Design review of the part built by this model. Coordinates are the model's own, in mm. Face numbers are marked on the shaded views. A direction names the side the tool comes from. Give positions to 0.01 mm unless a question says otherwise; leave off trailing zeros. Write each loop counter-clockwise with the first axis right and the second up, starting at its lowest first coordinate (ties: lowest second). Pieces come first, ordered by that corner, then holes. Notation, with made-up numbers: (34, 17) -> (81, 17) arc R31 cw to (81, 46) -> close; hole circle Ø9 at (53.5, 12.25). An arc over 180 degrees is marked (long way). Answer as a JSON object with one key per item and string values.
```python
from build123d import *

# Parameters (mm, degrees)
ESQUISSE1_R             = 3.65
BOSS_EXTRU_1_DEPTH      = 7.5
ESQUISSE2_R             = 1.45
ENL_V_MAT_EXTRU_1_DEPTH = 7.2
ENL_V_MAT_EXTRU_1_DRAFT = -0.5
ESQUISSE3_R             = 2.1
BOSS_EXTRU_2_DEPTH      = 5
BOSS_EXTRU_2_DRAFT      = -1
CONG_2_R                = 0.5


with BuildPart() as part:
    # Esquisse1 → Boss.-Extru.1 (new body)
    with BuildSketch(Plane.XY):
        Circle(ESQUISSE1_R)
    extrude(amount=BOSS_EXTRU_1_DEPTH)


with BuildPart() as enl_v_mat_extru_1_tool:
    # Esquisse2 → Enlèv. mat.-Extru.1 (with draft: the straight prism first)
    with BuildSketch(Plane(origin=(4, 0, 0), x_dir=(0, 0, -1), z_dir=(1, 0, 0))):
        with Locations((-3, 0)):
            Circle(ESQUISSE2_R)
    extrude(amount=-ENL_V_MAT_EXTRU_1_DEPTH)
    # Enlèv. mat.-Extru.1: the draft: its side faces are tilted about the plane it starts from
    enl_v_mat_extru_1_sides = [enl_v_mat_extru_1_tool.faces().sort_by_distance(p)[0] for p in [
        (0.4, 0, 4.45),
    ]]
    draft(enl_v_mat_extru_1_sides, Plane(origin=(4, 0, 0), x_dir=(0, 0, -1), z_dir=(1, 0, 0)), ENL_V_MAT_EXTRU_1_DRAFT)


with BuildPart() as part_1:
    add(part.part)

    # Enlèv. mat.-Extru.1: cut by enl_v_mat_extru_1_tool
    add(enl_v_mat_extru_1_tool.part, mode=Mode.SUBTRACT)


with BuildPart() as boss_extru_2_tool:
    # Esquisse3 → Boss.-Extru.2 (with draft: the straight prism first)
    with BuildSketch(Plane.XY.offset(7.5)):
        Circle(ESQUISSE3_R)
    extrude(amount=BOSS_EXTRU_2_DEPTH)
    # Boss.-Extru.2: the draft: its side faces are tilted about the plane it starts from
    boss_extru_2_sides = [boss_extru_2_tool.faces().sort_by_distance(p)[0] for p in [
        (-2.1, 0, 10),
    ]]
    draft(boss_extru_2_sides, Plane.XY.offset(7.5), BOSS_EXTRU_2_DRAFT)


with BuildPart() as part_2:
    add(part_1.part)

    # Boss.-Extru.2: add boss_extru_2_tool
    add(boss_extru_2_tool.part)

    # Congé2
    cong_2_edges = [part_2.edges().sort_by_distance(p)[0] for p in [
        (-2.1, 0, 7.5),
        (-2.187275325, 0, 12.5),
        (-3.65, 0, 0),
        (-3.65, 0, 7.5),
    ]]
    fillet(cong_2_edges, radius=CONG_2_R)


solid = part_2.part
```
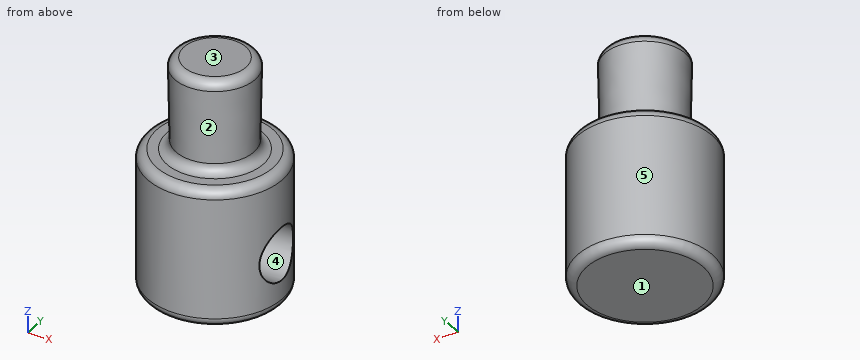
(1) For line 1 along Z through (x, y) = (2.5, -1.5); line 2 along Z through (x, y) = (-2, -0.25); line 3 along Z through (x, y) = (2.75, 0), list the stretches that pass through material, from the lowest coordinate up.
Here are the results:
{"line 1": "z = 0 to 7.5", "line 2": "z = 0 to 1.62, 4.38 to 12.37", "line 3": "z = 0 to 1.56, 4.44 to 7.5"}
(2) We need section A-A, the plane z = 7.25. State the section outline as (x, y) points, then the cut area to 3 significant figures.
Here are the results:
{"outline": "circle Ø7.17 at (0, 0)", "area": "40.3 mm²"}
(3) Clearance check with flat-ended pins moving along their axes: pin 1 (1 mm diameter, centred on x = -3, z = 3.5, fed in from +Y); pin 2 (3 mm diameter, centred on x = -1.5, y = 1.5, fed in from +Z); pin 3 (3 mm diameter, centred on y = -0.5, z = 11, fed in from -X); pin 4 (2 mm diameter, centred on y = 0.5, z = 3, fed in from +X). State where each tip first meets the part, or that it passes through.
Here are the results:
{"pin 1": "stops at y = 2.66", "pin 2": "stops at z = 12.5", "pin 3": "stops at x = -2.18", "pin 4": "stops at x = 3.4"}
(4) For the marked faces 4 and 5, list the 3-axis set-ups (+Z, -Z, +X, -X, +Y, -Y) from which the entire face can be reached by the end or side of a thin tool; tool diameter is ignored.
Here are the results:
{"face 4": "+X", "face 5": "+Z, -Z"}
(5) The part is to be moulded in two halves that separate along Z. For the marked faces 1, 2 and 3, say which applies: +Z half, -Z half, draft (parallel to the pull), parting line (faces both ways), or undercut.
Here are the results:
{"face 1": "-Z half", "face 2": "undercut", "face 3": "+Z half"}
